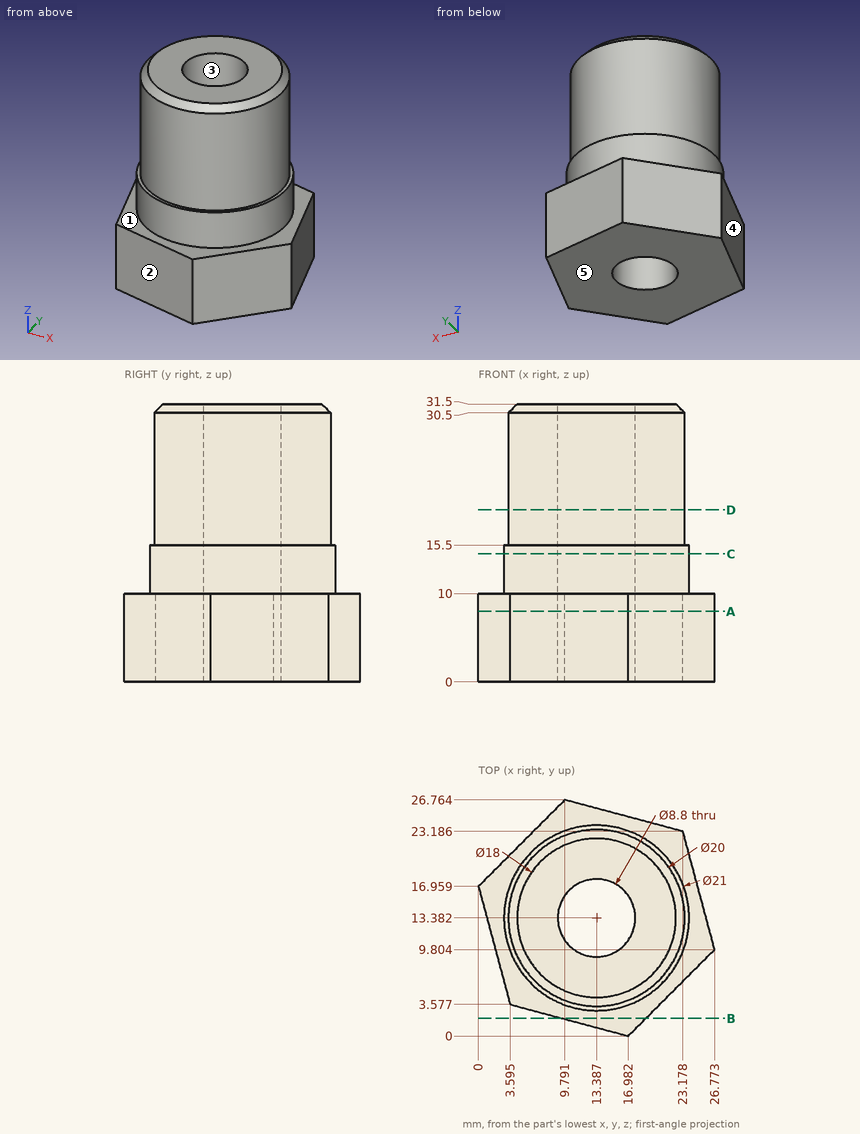
Print and shaded views of the part. All mm, measured from the part's lowest x, y and z. A direction names the side the tool comes from. Round coordinates to 2 decimals unless told otherwise and drop trailing zeros. Write each loop counter-clockwise with the first axis right and the second up, starting at its lowest first coordinate (ties: lowest second). Pieces come first, ordered by that corner, then holes. Notation, with made-up numbers: (40.25, 85) - (93.25, 85) arc R23 ccw to (93.25, 108) - close; hole circle Ø8 at (38.25, 23.5). An arc over 180 degrees is marked (long way). One line per item, written item: value.
(1) Cut at B-B, the plane y = 2. Give the cut face in (x, z).
Values follow:
outline: (9.5, 0) - (18.98, 0) - (18.98, 10) - (9.5, 10) - close
(2) Cut at A-A, the plane z = 8. Give the cut face in (x, y) (1 decimal).
Values follow:
outline: (0, 17) - (3.6, 3.6) - (17, 0) - (26.8, 9.8) - (23.2, 23.2) - (9.8, 26.8) - close; hole circle Ø8.8 at (13.4, 13.4)
(3) Cut at C-C, the plane z = 14.5. Give the cut face in (x, y).
Values follow:
outline: circle Ø21 at (13.39, 13.38); hole circle Ø8.8 at (13.39, 13.38)
(4) Drop flat-ended pins along their axis: P1, Ø12, axis at y = 4.5, z = 20.5, coming from the +X side; P2, Ø4, axis at y = 14.5, z = 15.5, coming from the +X side; P3, Ø6, axis at x = 19.5, z = 18.5, coming from the +Y side (1 decimal). Give the stop position or say it passes through.
Values follow:
P1: stops at x = 22.96
P2: stops at x = 23.89
P3: stops at y = 22.9
(5) Cut at D-D, the plane z = 19.5. Give the cut face in (x, y), plus the area to 3 significant figures.
Values follow:
outline: circle Ø20 at (13.39, 13.38); hole circle Ø8.8 at (13.39, 13.38)
area: 253 mm²
(6) Wall check: probe 1 along Z at (x, y) = (8.5, 25); probe 2 along Y at (x, z) = (12.25, 27.5); probe 3 along Z at (x, y) = (11.5, 3.25). Give the ranges that are in metal, low to high.
Values follow:
probe 1: z = 0 to 10
probe 2: y = 3.45 to 9.13, 17.63 to 23.32
probe 3: z = 0 to 15.5
(7) Two-plate mould, pull along Y, no slides. Class the marked faces 3, 4 and 5: pulls with the +Y half, pulls with the -Y half, needs draft (parallel to the pull), parting line crosses it, or undercut.
Values follow:
face 3: undercut
face 4: pulls with the -Y half
face 5: needs draft
(8) 3-axis set-ups, long thin cutter, end or side, ignore diameter. For the marked faces 1 and 2: which of +Z, -Z, +X, -X, +Y, -Y reach the whole face in a straight line?
Values follow:
face 1: +Z
face 2: +Z, -Z, -X, -Y
